Geometry check sheet. Reference: the model listing, model coordinates, mm. Face numbers are marked on the shaded views. A direction names the side the tool comes from. Round coordinates to 2 decimals unless told otherwise and drop trailing zeros. Write each loop counter-clockwise with the first axis right and the second up, starting at its lowest first coordinate (ties: lowest second). Pieces come first, ordered by that corner, then holes. Notation, with made-up numbers: M 15,25.5 L 24,25.5 A36 ccw 24,64.5 Z; hole C 21,1 d11. An arc over 180 degrees is marked long. One line per item, written item: value. Start each with the question number.
1. Scan lines: probe 1 along Y at (x, z) = (-1.45, 0.5); probe 2 along Z at (x, y) = (-0.1, 23.5); probe 3 along Z at (x, y) = (-1.05, 31). Record each from-to range of solid material in increasing order. Write a range as [from, to].
2. Section check A-A (y = 6). Record the boundary of the cut face in (x, z).
3. Depth check by flat-ended pin: P1, Ø1.5, axis at x = 0, y = 22, coming from the -Z side. Enter the tip coordinate at first touch or a pass-through.
4. Access from +Z, -Z, +X, -X, +Y, -Y to the whole of each face (thin tool, end or side, straight path). Record for the marked faces 1 and 2.
from build123d import *

# Parameters (mm, degrees)
F0_R     = 1.5
F1_DEPTH = 40
F2_R     = 3
F3_DEPTH = 2
F4_R     = 1.5
F5_R     = 0.49999


# Not quite as in the source:
# - a fillet or chamfer is up to 0.001 mm smaller than in the source, because OpenCascade refuses the exact size


with BuildPart() as f1:
    # F0 (on Front) → F1 (new body)
    with BuildSketch(Plane.XZ):
        Circle(F0_R)
    extrude(amount=-F1_DEPTH)

    # F2 (on face) → F3 (join)
    with BuildSketch(Plane.XZ):
        Circle(F2_R)
    extrude(amount=F3_DEPTH)

    # F4
    f4_edges = [f1.edges().sort_by_distance(p)[0] for p in [
        (-3, -2, 0),
    ]]
    fillet(f4_edges, radius=F4_R)

    # F5 (radius 0.5 in the source; OpenCascade refuses exactly that, so slightly less here)
    f5_edges = [f1.edges().sort_by_distance(p)[0] for p in [
        (-3, 0, 0),
    ]]
    fillet(f5_edges, radius=F5_R)


solid = f1.part
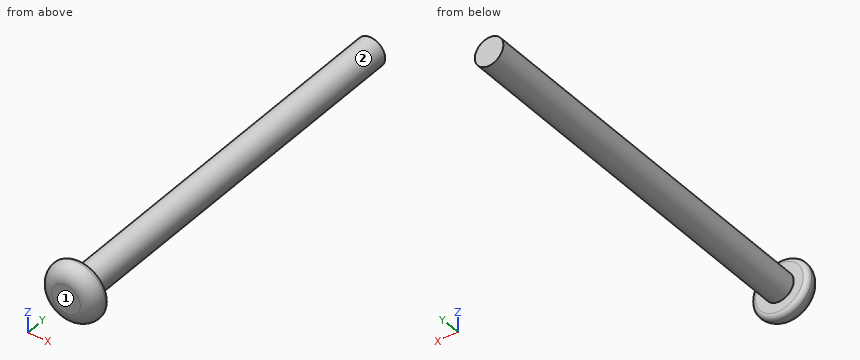
Result sheet:
1. probe 1: y = [-2, 0]
1. probe 2: z = [-1.5, 1.5]
1. probe 3: z = [-1.07, 1.07]
2. outline: C 0,0 d3
3. P1: stops at z = -1.5
4. face 1: +Z, -Z, +X, -X, -Y
4. face 2: +Y
